Here's how the part is built. I have some questions about the finished solid (model axes, mm). A direction names the side the tool comes from. Round coordinates to 2 decimals unless told otherwise and drop trailing zeros. Write each loop counter-clockwise with the first axis right and the second up, starting at its lowest first coordinate (ties: lowest second). Pieces come first, ordered by that corner, then holes. Notation, with made-up numbers: (-25.75, 36.25) - (-5.75, 36.25) arc R22 ccw to (-5.75, 47.25) - close; hole circle Ø8 at (-36.75, 52). An arc over 180 degrees is marked (long way). Return JSON: item names as keys, results as strings. Group by question number.
```python
from build123d import *

# Parameters (mm, degrees)
CHAMFER_1_SIZE  = 0.3
CHAMFER_2_SIZE  = 1
CHAMFER_2_SIZE2 = 0.3


with BuildPart() as part:
    # ｽｹｯﾁ1 → 回転1 (revolve)
    with BuildSketch(Plane.XY, mode=Mode.PRIVATE) as revolve_1_sk:
        Polygon((0, 3), (0, 6), (-1, 6), (-1, 4), (-11, 4), (-11, 3), align=None)
    revolve(revolve_1_sk.sketch.rotate(Axis((0, 0, 0), (1, 0, 0)), 90), axis=Axis((0, 0, 0), (1, 0, 0)))

    # 面取り1
    chamfer_1_edges = [part.edges().sort_by_distance(p)[0] for p in [
        (0, 0, -3),
    ]]
    chamfer(chamfer_1_edges, length=CHAMFER_1_SIZE)

    # 面取り2
    chamfer_2_edges = [part.edges().sort_by_distance(p)[0] for p in [
        (-11, 0, -4),
    ]]
    chamfer_2_side = [part.faces().sort_by_distance(p)[0] for p in [
        (-6, 0, -4),
    ]]
    chamfer(chamfer_2_edges, length=CHAMFER_2_SIZE, length2=CHAMFER_2_SIZE2, reference=chamfer_2_side[0])


solid = part.part
```
1) Will these pins go through, and if not, where does the flat tip stop? pin 1 Ø5 at (x, z) = (-9.5, 2.5) entering from -Y; pin 2 Ø5 at (x, y) = (-9, -3.5) entering from -Z; pin 3 Ø3 at (y, z) = (1, 0) entering from -X.
2) For faces 1 (the flat face through (-1, 3.92, -1.42)), 2 (the flat face through (0, 3, -3)), which set-ups out of +Z, -Z, +X, -X, +Y, -Y let a thin tool reach every point of the face, with its end or its side?
3) Imagine slicing it at C-C (x = -2.5). Please give me the cut outline in (y, z), plus the area to 3 significant figures.
4) If we mould it in two halves opening along Z, with no side actions, what happens to faces 3 (the cylindrical face through (-0.507, -1.802, 5.723)), 4 (the flat face through (-11, -3, -1)), 5 (the cylindrical face through (-5.58, -0.9, 2.86))? For each: released by +Z, released by -Z, zero draft, split by the parting line, or undercut.
5) Imagine slicing it at A-A (y = 0). Please give me the cut outline in (x, z), plus the area to 3 significant figures.
6) I need wall thicknesses on line 1 along Y through (x, z) = (-5.25, 0); line 2 along Z through (x, y) = (-10.5, -2.25); line 3 along Z through (x, y) = (-4.5, -0.75). Which ranges of each line are inside material? Lowest first, please.
7) Imagine slicing it at D-D (y = -4.75). Please give me the cut outline in (x, z).
Results found:
{
 "1": {"pin 1": "stops at y = -4", "pin 2": "stops at z = -3.87", "pin 3": "passes through"},
 "2": {"face 1": "-X", "face 2": "+Z, -Z, +X, +Y, -Y"},
 "3": {"outline": "circle Ø8 at (0, 0); hole circle Ø6 at (0, 0)", "area": "22.0 mm²"},
 "4": {"face 3": "split by the parting line", "face 4": "zero draft", "face 5": "undercut"},
 "5": {"outline": "(-11, -3.7) - (-10, -4) - (-1, -4) - (-1, -6) - (0, -6) - (0, -3.3) - (-0.3, -3) - (-11, -3) - close; (-11, 3) - (-0.3, 3) - (0, 3.3) - (0, 6) - (-1, 6) - (-1, 4) - (-10, 4) - (-11, 3.7) - close", "area": "25.6 mm²"},
 "6": {"line 1": "y = -4 to -3, 3 to 4", "line 2": "z = -3.12 to -1.98, 1.98 to 3.12", "line 3": "z = -3.93 to -2.9, 2.9 to 3.93"},
 "7": {"outline": "(-1, -3.67) - (0, -3.67) - (0, 3.67) - (-1, 3.67) - close"}
}
